Could you check a few things on this model? Use its own coordinates, in mm. A direction names the side the tool comes from. Round coordinates to 2 decimals unless told otherwise and drop trailing zeros. Write each loop counter-clockwise with the first axis right and the second up, starting at its lowest first coordinate (ties: lowest second). Pieces come first, ordered by that corner, then holes. Notation, with made-up numbers: (48.25, 77) - (81.25, 77) arc R25 ccw to (81.25, 110) - close; hole circle Ø8 at (86, -8). An arc over 180 degrees is marked (long way). Put each result on its own line as item: value.
from build123d import *

# Parameters (mm, degrees)
SKETCH1_R      = 4.064
SKETCH1_R_2    = 1.143
SKETCH1_R_3    = 2.1844
EXTRUDE2_DEPTH = 1.5748
SKETCH3_W      = 7.9502
SKETCH3_H      = 1.5748
SKETCH3_W_2    = 41.2496
EXTRUDE3_DEPTH = 22.6314
FILLET1_R      = 3.175
FILLET2_R      = 1.5748
FILLET3_R      = 0.254
SKETCH4_R      = 1.143
EXTRUDE4_DEPTH = 1.5748
SKETCH5_R      = 2.1844
EXTRUDE5_DEPTH = 1.5748


with BuildPart() as part:
    # Sketch1 → Extrude2 (new body)
    with BuildSketch(Plane.XY):
        with BuildLine():
            Line((11.9126, 30.734), (11.9126, 34.835994844))
            ThreePointArc((11.9126, 34.835994844), (12.84253597, 37.081058874), (15.0876, 38.010994844))
            Line((15.0876, 38.010994844), (43.6626, 38.010994844))
            ThreePointArc((43.6626, 38.010994844), (45.90766403, 37.081058874), (46.8376, 34.835994844))
            Line((46.8376, 34.835994844), (46.8376, 33.528))
            Line((46.8376, 33.528), (46.8376, 25.4))
            Line((46.8376, 25.4), (49.9872, 25.4))
            Line((49.9872, 25.4), (49.9872, 33.528))
            Line((49.9872, 33.528), (57.9374, 33.528))
            Line((57.9374, 33.528), (57.9374, 13.716))
            ThreePointArc((57.9374, 13.716), (57.00746403, 11.47093597), (54.7624, 10.541))
            Line((54.7624, 10.541), (49.9872, 10.541))
            Line((49.9872, 10.541), (49.9872, 0))
            Line((49.9872, 0), (8.7376, 0))
            Line((8.7376, 0), (8.7376, 10.541))
            Line((8.7376, 10.541), (3.9624, 10.541))
            ThreePointArc((3.9624, 10.541), (1.71733597, 11.47093597), (0.7874, 13.716))
            Line((0.7874, 13.716), (0.7874, 33.528))
            Line((0.7874, 33.528), (8.7376, 33.528))
            Line((8.7376, 33.528), (8.7376, 25.4))
            Line((8.7376, 25.4), (11.9126, 25.4))
            Line((11.9126, 25.4), (11.9126, 30.734))
        make_face()
        with Locations((21.0312, 22.8092)):
            Circle(SKETCH1_R, mode=Mode.SUBTRACT)
        with Locations((21.0312, 31.1912)):
            Circle(SKETCH1_R_2, mode=Mode.SUBTRACT)
        with Locations((29.4132, 22.8092)):
            Circle(SKETCH1_R_2, mode=Mode.SUBTRACT)
        with Locations((21.0312, 14.4272)):
            Circle(SKETCH1_R_2, mode=Mode.SUBTRACT)
        with Locations((12.6492, 22.8092)):
            Circle(SKETCH1_R_2, mode=Mode.SUBTRACT)
        with Locations((37.7952, 31.1912)):
            Circle(SKETCH1_R_2, mode=Mode.SUBTRACT)
        with Locations((46.1772, 22.8092)):
            Circle(SKETCH1_R_2, mode=Mode.SUBTRACT)
        with Locations((37.7952, 22.8092)):
            Circle(SKETCH1_R, mode=Mode.SUBTRACT)
        with Locations((37.7952, 14.4272)):
            Circle(SKETCH1_R_2, mode=Mode.SUBTRACT)
        with Locations((4.5466, 25.5778)):
            Circle(SKETCH1_R_3, mode=Mode.SUBTRACT)
        with Locations((4.5466, 15.7734)):
            Circle(SKETCH1_R_3, mode=Mode.SUBTRACT)
        with Locations((53.7464, 25.5778)):
            Circle(SKETCH1_R_3, mode=Mode.SUBTRACT)
        with Locations((53.7464, 15.7734)):
            Circle(SKETCH1_R_3, mode=Mode.SUBTRACT)
    extrude(amount=EXTRUDE2_DEPTH)

    # Sketch3 → Extrude3 (add)
    with BuildSketch(Plane.XY.offset(1.5748)):
        with Locations((4.7625, 32.7406)):
            Rectangle(SKETCH3_W, SKETCH3_H)
        with Locations((29.3624, 0.7874)):
            Rectangle(SKETCH3_W_2, SKETCH3_H)
        with Locations((53.9623, 32.7406)):
            Rectangle(SKETCH3_W, SKETCH3_H)
    extrude(amount=EXTRUDE3_DEPTH)

    # Fillet1
    fillet1_edges = [part.edges().sort_by_distance(p)[0] for p in [
        (0.7874, 32.7406, 24.2062),
        (8.7376, 0.7874, 24.2062),
        (49.9872, 0.7874, 24.2062),
        (57.9374, 32.7406, 24.2062),
    ]]
    fillet(fillet1_edges, radius=FILLET1_R)

    # Fillet2
    fillet2_edges = [part.edges().sort_by_distance(p)[0] for p in [
        (4.7625, 33.528, 0),
        (53.9623, 33.528, 0),
        (29.3624, 0, 0),
    ]]
    fillet(fillet2_edges, radius=FILLET2_R)

    # Fillet3
    fillet3_edges = [part.edges().sort_by_distance(p)[0] for p in [
        (4.7625, 31.9532, 1.5748),
        (29.3624, 1.5748, 1.5748),
        (53.9623, 31.9532, 1.5748),
    ]]
    fillet(fillet3_edges, radius=FILLET3_R)

    # Sketch4 → Extrude4 (cut)
    with BuildSketch(Plane.XZ):
        with Locations(Location((19.6342, 14.2494, 0), (0, 0, 270))):
            Circle(SKETCH4_R)
        with Locations(Location((38.6588, 14.2494, 0), (0, 0, 270))):
            Circle(SKETCH4_R)
    extrude(amount=-EXTRUDE4_DEPTH, mode=Mode.SUBTRACT)

    # Sketch5 → Extrude5 (cut)
    with BuildSketch(Plane(origin=(0, 33.528, 0), x_dir=(1, 0, 0), z_dir=(0, 1, 0))):
        with Locations(Location((4.5466, -9.3218, 0), (0, 0, 270))):
            Circle(SKETCH5_R)
        with Locations(Location((4.5466, -19.1262, 0), (0, 0, 270))):
            Circle(SKETCH5_R)
        with Locations(Location((53.7464, -19.1262, 0), (0, 0, 270))):
            Circle(SKETCH5_R)
        with Locations(Location((53.7464, -9.3218, 0), (0, 0, 270))):
            Circle(SKETCH5_R)
    extrude(amount=-EXTRUDE5_DEPTH, mode=Mode.SUBTRACT)


solid = part.part
(1) For faces 1 (the face through (29, 1.575, 13)), 2 (the face through (4.818, 33.079, 0.474)), 3 (the face through (6, 10.541, 1)), which set-ups out of +Z, -Z, +X, -X, +Y, -Y let a thin tool reach every point of the face, with its end or its side?
Values found:
face 1: +Z, +X, -X, +Y
face 2: -Z, -X, +Y
face 3: +Z, -Z, -X, -Y
(2) I'm going to push flat-ended pins straight in: pin 1 (5 mm diameter, centred on x = 4.55, z = 19.13, fed in from +Y); pin 2 (3 mm diameter, centred on x = 43, z = 4.5, fed in from +Y); pin 3 (3 mm diameter, centred on x = 21.03, y = 31.19, fed in from +Z). Where does each tip first touch, or does it pass through?
Values found:
pin 1: stops at y = 33.53
pin 2: stops at y = 1.57
pin 3: stops at z = 1.57
(3) If we mould it in two halves opening along X, with no side actions, what happens to faces 4 (the face through (45.88, 37.11, 0.78)), 5 (the face through (5, 31.953, 13)), 6 (the face through (6.39, 32.75, 20.3)), 7 (the face through (33.735, 22.988, 0.776))? For each: pulls with the +X half, pulls with the -X half, needs draft (parallel to the pull), parting line crosses it, or undercut.
Values found:
face 4: pulls with the +X half
face 5: needs draft
face 6: undercut
face 7: undercut
(4) Imagine slicing it at B-B, the plane x = 27. List the corners of the cut face in (y, z) for me.
Values found:
outline: (0, 1.57) arc R1.57 ccw to (1.57, 0) - (38.01, 0) - (38.01, 1.57) - (1.83, 1.57) arc R0.25 cw to (1.57, 1.83) - (1.57, 24.21) - (0, 24.21) - close
(5) Imagine slicing it at D-D, the plane y = 7.5. List the corners of the cut face in (x, z) for me, then the cut area to 3 significant figures.
Values found:
outline: (8.74, 0) - (49.99, 0) - (49.99, 1.57) - (8.74, 1.57) - close
area: 65.0 mm^2
(6) Please list where these lines run through material, in increasing order: probe 1 along X at (y, z) = (32, 5); probe 2 along Y at (x, z) = (27, 15.5). Write a range as from..to.
Values found:
probe 1: x = 0.79..8.74, 49.99..57.94
probe 2: y = 0..1.57
(7) Imagine slicing it at C-C, the plane x = 40.5. List the corners of the cut face in (y, z) for me, then the cut area to 3 significant figures.
Values found:
outline: (0, 1.57) arc R1.57 ccw to (1.57, 0) - (19.78, 0) - (19.78, 1.57) - (1.83, 1.57) arc R0.25 cw to (1.57, 1.83) - (1.57, 24.21) - (0, 24.21) - close; (25.84, 0) - (38.01, 0) - (38.01, 1.57) - (25.84, 1.57) - close
area: 85.4 mm^2
(8) Imagine slicing it at A-A, the plane z = 10.5. List the corners of the cut face in (x, y) for me.
Values found:
outline: (0.79, 31.95) - (2.71, 31.95) - (2.71, 33.53) - (0.79, 33.53) - close; (6.39, 31.95) - (8.74, 31.95) - (8.74, 33.53) - (6.39, 33.53) - close; (8.74, 0) - (49.99, 0) - (49.99, 1.57) - (8.74, 1.57) - close; (49.99, 31.95) - (51.91, 31.95) - (51.91, 33.53) - (49.99, 33.53) - close; (55.59, 31.95) - (57.94, 31.95) - (57.94, 33.53) - (55.59, 33.53) - close
